```python
from build123d import *

# Parameters (mm, degrees)
SKETCH1_R           = 8
SKETCH1_R_2         = 1.5
BOSS_EXTRUDE1_DEPTH = 2.2
BOSS_EXTRUDE2_START = 2.2
SKETCH1_3_R         = 8
SKETCH1_3_R_2       = 4
BOSS_EXTRUDE2_DEPTH = 3
FILLET1_R           = 7
CUT_EXTRUDE2_START  = -5.2
SKETCH2_R           = 8.05
SKETCH2_R_2         = 7
CUT_EXTRUDE2_DEPTH  = 2.2
SKETCH2_4_R         = 7
SKETCH2_4_R_2       = 4
BOSS_EXTRUDE3_DEPTH = 2.2
BOSS_EXTRUDE4_START = 2.2
SKETCH2_5_R         = 7
SKETCH2_5_R_2       = 4
BOSS_EXTRUDE4_DEPTH = 2
FILLET2_START       = -35.2
FILLET2_2_DEPTH     = 4.2
SKETCH3_R           = 8.15
SKETCH3_R_2         = 8.05
CUT_EXTRUDE3_DEPTH  = 2.2


with BuildPart() as part:
    # Sketch1 → Boss-Extrude1 (new body)
    # profile 1 of 4: a face of its own
    with BuildSketch(Plane(origin=(0, 0, -25.8), x_dir=(-1, 0, 0), z_dir=(0, 0, -1))):
        Polygon((-133.135100578, -5.831793049), (-133.135100578, 6.168206951), (-159.569076944, 16.05794409), (-170.376148703, -4.244942404), (-164.993668486, -14.43595779), align=None)
        with Locations((-150, 0)):
            Circle(SKETCH1_R, mode=Mode.SUBTRACT)
        Polygon((-165.667996862, -6.414349097), (-164.131074119, -9.324309317), (-160.842513273, -9.448275288), (-159.09087517, -6.662281039), (-160.627797913, -3.752320819), (-163.916358759, -3.628354848), align=None, mode=Mode.SUBTRACT)
        Polygon((-140.417550289, 1.645448267), (-140.417550289, -1.645448267), (-137.567550289, -3.290896534), (-134.717550289, -1.645448267), (-134.717550289, 1.645448267), (-137.567550289, 3.290896534), align=None, mode=Mode.SUBTRACT)
        Polygon((-160.873796009, 9.464930151), (-158.542174952, 7.142529831), (-155.365106749, 8.000572737), (-154.519659602, 11.181015965), (-156.851280658, 13.503416285), (-160.028348862, 12.645373378), align=None, mode=Mode.SUBTRACT)
    # profile 2 of 4: a face of its own
    with BuildSketch(Plane(origin=(0, 0, -25.8), x_dir=(-1, 0, 0), z_dir=(0, 0, -1))):
        Polygon((-163.916358759, -3.628354848), (-165.667996862, -6.414349097), (-164.131074119, -9.324309317), (-160.842513273, -9.448275288), (-159.09087517, -6.662281039), (-160.627797913, -3.752320819), align=None)
        with Locations((-162.379436016, -6.538315068)):
            Circle(SKETCH1_R_2, mode=Mode.SUBTRACT)
    # profile 3 of 4: a face of its own
    with BuildSketch(Plane(origin=(0, 0, -25.8), x_dir=(-1, 0, 0), z_dir=(0, 0, -1))):
        Polygon((-160.028348862, 12.645373378), (-160.873796009, 9.464930151), (-158.542174952, 7.142529831), (-155.365106749, 8.000572737), (-154.519659602, 11.181015965), (-156.851280658, 13.503416285), align=None)
        with Locations((-157.696727805, 10.322973058)):
            Circle(SKETCH1_R_2, mode=Mode.SUBTRACT)
    # profile 4 of 4: a face of its own
    with BuildSketch(Plane(origin=(0, 0, -25.8), x_dir=(-1, 0, 0), z_dir=(0, 0, -1))):
        Polygon((-137.567550289, 3.290896534), (-140.417550289, 1.645448267), (-140.417550289, -1.645448267), (-137.567550289, -3.290896534), (-134.717550289, -1.645448267), (-134.717550289, 1.645448267), align=None)
        with Locations((-137.567550289, 0)):
            Circle(SKETCH1_R_2, mode=Mode.SUBTRACT)
    extrude(amount=BOSS_EXTRUDE1_DEPTH)

    # Sketch1<3> → Boss-Extrude2 (add)
    # profile 1 of 2: a face of its own
    with BuildSketch(Plane(origin=(0, 0, -25.8), x_dir=(-1, 0, 0), z_dir=(0, 0, -1)).offset(BOSS_EXTRUDE2_START)):
        Polygon((-133.135100578, -5.831793049), (-133.135100578, 6.168206951), (-159.569076944, 16.05794409), (-170.376148703, -4.244942404), (-164.993668486, -14.43595779), align=None)
        with Locations((-150, 0)):
            Circle(SKETCH1_3_R, mode=Mode.SUBTRACT)
        Polygon((-165.667996862, -6.414349097), (-164.131074119, -9.324309317), (-160.842513273, -9.448275288), (-159.09087517, -6.662281039), (-160.627797913, -3.752320819), (-163.916358759, -3.628354848), align=None, mode=Mode.SUBTRACT)
        Polygon((-140.417550289, 1.645448267), (-140.417550289, -1.645448267), (-137.567550289, -3.290896534), (-134.717550289, -1.645448267), (-134.717550289, 1.645448267), (-137.567550289, 3.290896534), align=None, mode=Mode.SUBTRACT)
        Polygon((-160.873796009, 9.464930151), (-158.542174952, 7.142529831), (-155.365106749, 8.000572737), (-154.519659602, 11.181015965), (-156.851280658, 13.503416285), (-160.028348862, 12.645373378), align=None, mode=Mode.SUBTRACT)
    # profile 2 of 2: a face of its own
    with BuildSketch(Plane(origin=(0, 0, -25.8), x_dir=(-1, 0, 0), z_dir=(0, 0, -1)).offset(BOSS_EXTRUDE2_START)):
        with Locations((-150, 0)):
            Circle(SKETCH1_3_R)
        with Locations((-150, 0)):
            Circle(SKETCH1_3_R_2, mode=Mode.SUBTRACT)
    extrude(amount=BOSS_EXTRUDE2_DEPTH)

    # Fillet1
    fillet1_edges = [part.edges().sort_by_distance(p)[0] for p in [
        (133.135100578, -5.831793049, -28.4),
        (164.993668486, -14.43595779, -28.4),
        (170.376148703, -4.244942404, -28.4),
        (159.569076944, 16.05794409, -28.4),
        (133.135100578, 6.168206951, -28.4),
    ]]
    fillet(fillet1_edges, radius=FILLET1_R)

    # Sketch2 → Cut-Extrude2 (cut)
    with BuildSketch(Plane(origin=(0, 0, -31), x_dir=(-1, 0, 0), z_dir=(0, 0, -1)).offset(CUT_EXTRUDE2_START)):
        with Locations(Location((-150, 0, 0), (0, 0, 180))):
            Circle(SKETCH2_R)
        with Locations((-150, 0)):
            Circle(SKETCH2_R_2, mode=Mode.SUBTRACT)
    extrude(amount=CUT_EXTRUDE2_DEPTH, mode=Mode.SUBTRACT)

    # Sketch2<4> → Boss-Extrude3 (add)
    with BuildSketch(Plane(origin=(0, 0, -31), x_dir=(-1, 0, 0), z_dir=(0, 0, -1))):
        with Locations(Location((-150, 0, 0), (0, 0, 180))):
            Circle(SKETCH2_4_R)
        with Locations(Location((-150, 0, 0), (0, 0, 180))):
            Circle(SKETCH2_4_R_2, mode=Mode.SUBTRACT)
    extrude(amount=BOSS_EXTRUDE3_DEPTH)

    # Sketch2<5> → Boss-Extrude4 (add)
    # profile 1 of 2: a face of its own
    with BuildSketch(Plane(origin=(0, 0, -31), x_dir=(-1, 0, 0), z_dir=(0, 0, -1)).offset(BOSS_EXTRUDE4_START)):
        with Locations(Location((-150, 0, 0), (0, 0, 180))):
            Circle(SKETCH2_5_R)
        with Locations(Location((-150, 0, 0), (0, 0, 180))):
            Circle(SKETCH2_5_R_2, mode=Mode.SUBTRACT)
    # profile 2 of 2: a face of its own
    with BuildSketch(Plane(origin=(0, 0, -31), x_dir=(-1, 0, 0), z_dir=(0, 0, -1)).offset(BOSS_EXTRUDE4_START)):
        with Locations(Location((-150, 0, 0), (0, 0, 180))):
            Circle(SKETCH2_5_R_2)
    extrude(amount=BOSS_EXTRUDE4_DEPTH)

    # Fillet2: read off the stored shape, not the designer's step
    # Fillet2 outline → Fillet2 (revolve)
    with BuildSketch(Plane(origin=(150, 0, 0), x_dir=(1, 0, 0), z_dir=(0, -1, 0))):
        with BuildLine():
            ThreePointArc((7, -35.2), (9.58154807, -32.143379814), (13.415605973, -31))
            Line((13.415605973, -31), (7, -31))
            Line((7, -31), (7, -35.2))
        make_face()
    revolve(axis=Axis((150, 0, 0), (0, 0, 1)))

    # Fillet2 2 outline → Fillet2 2 (cut)
    with BuildSketch(Plane.XY.offset(FILLET2_START)):
        with BuildLine():
            Line((140.417550289, 1.645448267), (137.567550289, 3.290896534))
            Line((137.567550289, 3.290896534), (136.903212084, 2.907340693))
            ThreePointArc((136.903212084, 2.907340693), (136.584394027, 0), (136.903212084, -2.907340693))
            Line((136.903212084, -2.907340693), (137.567550289, -3.290896534))
            Line((137.567550289, -3.290896534), (140.417550289, -1.645448267))
            Line((140.417550289, -1.645448267), (140.417550289, 1.645448267))
        make_face()
        with BuildLine():
            Line((159.09087517, -6.662281039), (160.303741962, -8.59135526))
            ThreePointArc((160.303741962, -8.59135526), (161.862688268, -6.265389906), (162.904858589, -3.666484475))
            Line((162.904858589, -3.666484475), (160.627797913, -3.752320819))
            Line((160.627797913, -3.752320819), (159.09087517, -6.662281039))
        make_face()
        with BuildLine():
            Line((155.989734556, -12.004231069), (138.781383409, -7.356706152))
            ThreePointArc((138.781383409, -7.356706152), (146.50211867, -12.951575573), (155.989734556, -12.004231069))
        make_face()
        with BuildLine():
            ThreePointArc((152.074956497, 13.254170633), (145.29905415, 12.565014594), (139.734777095, 8.637342318))
            Line((139.734777095, 8.637342318), (152.074956497, 13.254170633))
        make_face()
        with BuildLine():
            Line((155.365106749, 8.000572737), (158.542174952, 7.142529831))
            Line((158.542174952, 7.142529831), (160.163207231, 8.7571515))
            ThreePointArc((160.163207231, 8.7571515), (158.046418581, 10.7346929), (155.554467123, 12.211731188))
            Line((155.554467123, 12.211731188), (154.519659602, 11.181015965))
            Line((154.519659602, 11.181015965), (155.365106749, 8.000572737))
        make_face()
    extrude(amount=FILLET2_2_DEPTH, mode=Mode.SUBTRACT)

    # Sketch3 → Cut-Extrude3 (cut)
    with BuildSketch(Plane.XY.offset(-25.8)):
        with Locations((150, 0)):
            Circle(SKETCH3_R)
        with Locations((150, 0)):
            Circle(SKETCH3_R_2, mode=Mode.SUBTRACT)
    extrude(amount=-CUT_EXTRUDE3_DEPTH, mode=Mode.SUBTRACT)


with BuildPart() as body_2:
    # Mirror3: mirrored copy
    add(part.part.mirror(Plane.ZX))


solid = body_2.part
```
Input: part model. Units: mm. Frame: model coordinates. A direction names the side the tool comes from. Give positions to 0.01 mm unless a question says otherwise; leave off trailing zeros. Loops run counter-clockwise (first coordinate to the right, second up) from the corner with the lowest first, then second, coordinate; pieces in that order, holes last. Notation, with made-up numbers: M 71.5,-14.75 L 98.5,-14.75 A31 cw 98.5,17.25 Z; hole C 55,-32 d6. An arc over 180 degrees is marked long. Answer as CSV lines item,"result". Start each with the question number.
1. Pin query (flat end, axial travel): P1, Ø5, axis at y = 4, z = -31.5, coming from the -X side; P2, Ø5, axis at x = 162.38, y = 6.54, coming from the -Z side; P3, Ø8.5, axis at x = 164, y = 1, coming from the -Z side. Return the tip coordinate at first contact, or that it passes through.
2. Reachability of faces 1 (the face through (159.87, 5.19, -29.71)), 2 (the face through (141.858, -0.358, -26.885)), 3 (the face through (160.994, 7.113, -26.885)) from +Z, -Z, +X, -X, +Y, -Y: full face, straight path, thin tool, end or side. Return the list, or none.
3. Section C-C on z = -26.75. Return loops of the section in (x, y).
4. Section B-B on z = -32.75. Return loops of the section in (x, y).
5. Pull-direction query (X, two-part tool) for faces 4 (the face through (150, 0, -33.2)), 5 (the face through (158.82, -13.87, -28.44)), 6 (the face through (134, -1, -31)); classes: released by +X, released by -X, zero draft, split by the parting line, or undercut.
6. Section D-D on z = -34.5. Return loops of the section in (x, y), plus the area to 3 significant figures.
7. Section A-A on z = -29.5. State how many separate pieces and enclosed holes the cut face has, plus the area to 3 significant figures.
8. Line query: L1, parallel to X at y = 0, z = -30.3; L2, parallel to X at y = 0, z = -27.2; L3, parallel to Z at x = 147, y = 5.5. Output: solid intervals per line, ascending.
Computed values:
1,P1,"stops at x = 133.22"
1,P2,"stops at z = -28"
1,P3,"stops at z = -32.01"
2,face 1,"-Z"
2,face 2,"+Z"
2,face 3,"+Z, -Z"
3,outline,"M 133.14,-1.31 A7 ccw 137.68,-7.87 L 153.82,-13.91 A7 ccw 162.45,-10.64 L 168.63,0.97 A7 ccw 168.64,7.53 L 167.61,9.49 A7 ccw 159.59,12.98 L 138.31,7.23 A7 ccw 133.14,0.47 Z; hole C 137.57,0 d3; hole C 150,0 d16.3; hole C 157.7,-10.32 d3; hole C 162.38,6.54 d3"
4,outline,"C 150,0 d17.57; hole C 150,0 d8"
5,face 4,"undercut"
5,face 5,"split by the parting line"
5,face 6,"zero draft"
6,outline,"C 150,0 d14.71"
6,area,"170 mm²"
7,separate pieces,"1"
7,enclosed holes,"4"
7,area,"570 mm²"
8,L1,"x = 133.14 to 134.72, 140.42 to 146, 154 to 168.12"
8,L2,"x = 133.14 to 136.07, 139.07 to 141.85, 158.15 to 168.12"
8,L3,"z = -35.2 to -28"
